```python
from build123d import *

# Parameters (mm, degrees)
F0_R       = 2.95
F1_DEPTH   = 22
F2_SIZE2   = 1.5
F2_SIZE    = 0.5
F2_2_SIZE2 = 1.5
F2_2_SIZE  = 0.5
F3_R       = 0.5


with BuildPart() as f1:
    # F0 (on Front) → F1 (new body)
    with BuildSketch(Plane.XZ):
        Circle(F0_R)
    extrude(amount=-F1_DEPTH)

    # F2
    f2_edges = [f1.edges().sort_by_distance(p)[0] for p in [
        (-2.95, 0, 0),
    ]]
    f2_side = f1.faces().sort_by_distance((0, 0, 0))[0]
    chamfer(f2_edges, length=F2_SIZE, length2=F2_SIZE2, reference=f2_side)

    # F2#2
    f2_2_edges = [f1.edges().sort_by_distance(p)[0] for p in [
        (-2.95, 22, 0),
    ]]
    f2_2_side = f1.faces().sort_by_distance((0, 22, 0))[0]
    chamfer(f2_2_edges, length=F2_2_SIZE, length2=F2_2_SIZE2, reference=f2_2_side)

    # F3
    f3_edges = [f1.edges().sort_by_distance(p)[0] for p in [
        (-2.45, 0, 0),
        (-2.45, 22, 0),
        (-2.95, 1.5, 0),
        (-2.95, 20.5, 0),
    ]]
    fillet(f3_edges, radius=F3_R)


solid = f1.part
```
Input: part model. Units: mm. Frame: model coordinates. Give positions to 0.01 mm unless a question says otherwise; leave off trailing zeros. Write each loop counter-clockwise with the first axis right and the second up, starting at its lowest first coordinate (ties: lowest second). Pieces come first, ordered by that corner, then holes. Notation, with made-up numbers: (62, -12) - (68, -12) arc R27 cw to (68, 12) - close; hole circle Ø7 at (48.25, 13.5). An arc over 180 degrees is marked (long way). Write item = value, one per line. Start each with the question number.
1) Pin query (flat end, axial travel): pin 1 (3 mm diameter, centred on x = -1, y = 11, fed in from +Z). Return the tip coordinate at first contact, or that it passes through.
2) Material intervals for L1, parallel to Z at x = -0.15, y = 14.25; L2, parallel to X at y = 19.5, z = 1.45, sorted ascending. Write a range as [from, to].
3) Cut plane A-A (y = 10). Return loops of the section in (x, z).
Answers follow:
q1.pin_1 = 2.95
q2.L1 = [-2.95, 2.95]
q2.L2 = [-2.57, 2.57]
q3.outline = circle Ø5.9 at (0, 0)
